```python
from build123d import *

# Parameters (mm, degrees)
SKETCH1_W           = 250
SKETCH1_H           = 300
SKETCH1_R           = 20
SKETCH1_R_2         = 51
BOSS_EXTRUDE1_DEPTH = 15
BOSS_EXTRUDE2_DEPTH = 15


with BuildPart() as part:
    # Sketch1 → Boss-Extrude1 (new body)
    with BuildSketch(Plane.XY):
        with Locations((-125, 150)):
            Rectangle(SKETCH1_W, SKETCH1_H)
        with Locations((-125, 230)):
            Circle(SKETCH1_R, mode=Mode.SUBTRACT)
        with Locations((-125, 150)):
            Circle(SKETCH1_R, mode=Mode.SUBTRACT)
        with Locations((-180, 70)):
            Circle(SKETCH1_R_2, mode=Mode.SUBTRACT)
        with Locations((-70, 70)):
            Circle(SKETCH1_R_2, mode=Mode.SUBTRACT)
    extrude(amount=BOSS_EXTRUDE1_DEPTH)

    # Sketch2 → Boss-Extrude2 (add)
    with BuildSketch(Plane.XY):
        Polygon((-190, 0), (-60, 0), (0, 0), (-60, -200), (-190, -200), (-250, 0), align=None)
    extrude(amount=BOSS_EXTRUDE2_DEPTH)


solid = part.part
```
Geometry: final body of the model. Coordinates: model frame, mm. Give positions to 0.01 mm unless a question says otherwise; leave off trailing zeros. Write each loop counter-clockwise with the first axis right and the second up, starting at its lowest first coordinate (ties: lowest second). Pieces come first, ordered by that corner, then holes.
1. Line query: probe 1 along Y at (x, z) = (-125, 7.75); probe 2 along X at (y, z) = (32, 5.25); probe 3 along Y at (x, z) = (-180, 8.5). Output: solid intervals per line, ascending.
2. Section query B-B, the plane x = -70. Return loops of the section in (y, z), then the cut area to 3 significant figures.
3. Section query C-C, the plane x = -175. Return loops of the section in (y, z).
4. Section query A-A, the plane y = 70. Return loops of the section in (x, z).
5. Section query D-D, the plane y = -152.5. Return loops of the section in (x, z).
6. Draft query along X for faces 1 (the flat face through (-123, 54, 15)), 2 (the cylindrical face through (-21.355, 85.319, 7.395)), 3 (the flat face through (-29.58, -98.6, 7.4)). Return one class per face: released by +X, released by -X, zero draft, split by the parting line, or undercut.
7. Pin query (flat end, axial travel): P1, Ø6, axis at y = -123, z = 6, coming from the +X side. Return the tip coordinate at first contact, or that it passes through.
Computed:
1. probe 1: y = -200 to 130, 170 to 210, 250 to 300
1. probe 2: x = -250 to -214.01, -145.99 to -104.01, -35.99 to 0
1. probe 3: y = -200 to 19, 121 to 300
2. outline: (-200, 0) - (19, 0) - (19, 15) - (-200, 15) - close; (121, 0) - (300, 0) - (300, 15) - (121, 15) - close
2. area: 5,970 mm2
3. outline: (-200, 0) - (19.25, 0) - (19.25, 15) - (-200, 15) - close; (120.75, 0) - (300, 0) - (300, 15) - (120.75, 15) - close
4. outline: (-250, 0) - (-231, 0) - (-231, 15) - (-250, 15) - close; (-129, 0) - (-121, 0) - (-121, 15) - (-129, 15) - close; (-19, 0) - (0, 0) - (0, 15) - (-19, 15) - close
5. outline: (-204.25, 0) - (-45.75, 0) - (-45.75, 15) - (-204.25, 15) - close
6. face 1: zero draft
6. face 2: undercut
6. face 3: released by +X
7. P1: stops at x = -36
